Design review of the part shown in the three views and the two pictorial views. Dimensions are in mm from the part's minimum x, y and z. Round coordinates to 2 decimals unless told otherwise and drop trailing zeros. Write each loop counter-clockwise with the first axis right and the second up, starting at its lowest first coordinate (ties: lowest second). Pieces come first, ordered by that corner, then holes. Notation, with made-up numbers: (72.5, 0.5) -> (108.5, 0.5) arc R19 ccw to (108.5, 37.5) -> close; hole circle Ø1 at (72.5, 13). An arc over 180 degrees is marked (long way). One line per question, with ' | ' between items. Start each with the question number.
1) Consider section A-A (y = 23.1). Give the boundary of the cut face in (x, z), then the cut area to 3 significant figures.
2) Consider section C-C (z = 8). Give the boundary of the cut face in (x, y).
3) Consider section B-B (x = 9). Give the boundary of the cut face in (y, z).
4) Mouldability with a two-part tool opening along X and no side actions: class the marked faces 1, 2 and 3 as +X half, -X half, draft (parallel to the pull), parting line (faces both ways), or undercut.
5) Consider section D-D (x = 6). Give the boundary of the cut face in (y, z), then the cut area to 3 significant figures.
6) For probe 1 along Y at (x, z) = (9, 12.5); probe 2 along Y at (x, z) = (15.5, 8.5); probe 3 along Y at (x, z) = (3.75, 8.75), list the stretches that pass through material, from the lowest coordinate up.
7) Insertion check: pin 1 Ø1.5 at (x, z) = (13.5, 4.5) entering from -Y; pin 2 Ø1.1 at (x, y) = (8, 22.5) entering from -Z; pin 3 Ø1 at (x, z) = (14.5, 12.5) entering from +Y. Each pin has a flat end and moves straight along its axis. Give the tip position at first contact, or say it passes through.
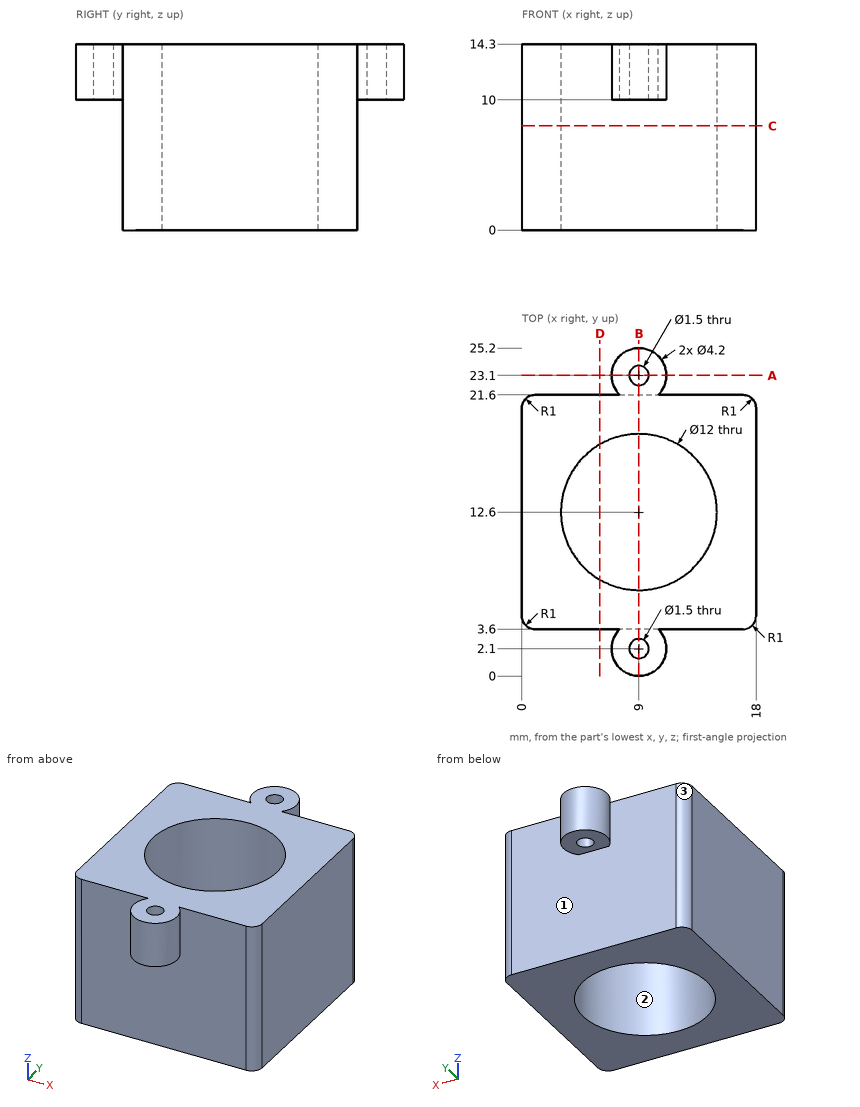
From the geometry:
1) outline: (6.9, 10) -> (8.25, 10) -> (8.25, 14.3) -> (6.9, 14.3) -> close; (9.75, 10) -> (11.1, 10) -> (11.1, 14.3) -> (9.75, 14.3) -> close | area: 11.6 mm2
2) outline: (0, 4.6) arc R1 ccw to (1, 3.6) -> (17, 3.6) arc R1 ccw to (18, 4.6) -> (18, 20.6) arc R1 ccw to (17, 21.6) -> (1, 21.6) arc R1 ccw to (0, 20.6) -> close; hole circle Ø12 at (9, 12.6)
3) outline: (0, 10) -> (1.35, 10) -> (1.35, 14.3) -> (0, 14.3) -> close; (2.85, 10) -> (3.6, 10) -> (3.6, 0) -> (6.6, 0) -> (6.6, 14.3) -> (2.85, 14.3) -> close; (18.6, 0) -> (21.6, 0) -> (21.6, 10) -> (22.35, 10) -> (22.35, 14.3) -> (18.6, 14.3) -> close; (23.85, 10) -> (25.2, 10) -> (25.2, 14.3) -> (23.85, 14.3) -> close
4) face 1: draft | face 2: undercut | face 3: -X half
5) outline: (3.6, 0) -> (7.4, 0) -> (7.4, 14.3) -> (3.6, 14.3) -> close; (17.8, 0) -> (21.6, 0) -> (21.6, 14.3) -> (17.8, 14.3) -> close | area: 109 mm2
6) probe 1: y = 0 to 1.35, 2.85 to 6.6, 18.6 to 22.35, 23.85 to 25.2 | probe 2: y = 3.6 to 21.6 | probe 3: y = 3.6 to 9.7, 15.5 to 21.6
7) pin 1: stops at y = 3.6 | pin 2: stops at z = 10 | pin 3: stops at y = 21.6
